Autodesk Inventor part; units mm, degrees
ref_plane "YZ Plane" through (0, 0, 0) normal (1, 0, 0) x (0, 1, 0)
ref_plane "XZ Plane" through (0, 0, 0) normal (0, 1, 0) x (-1, 0, 0)
ref_plane "XY Plane" through (0, 0, 0) normal (0, 0, 1) x (1, 0, 0)
sketch "Sketch1" plane through (0, 0, 0) normal (0, 0, 1) x (1, 0, 0)
  line L0 (0, 0) -> (5, 0)
  line L1 (5, 0) -> (5, 22)
  line L2 (5, 22) -> (0, 22)
  line L3 (0, 22) -> (0, 0)
  line L4 (2.5, 0) -> (2.5, 22) construction
  circle A0 centre (2.5, 13.75) radius 1.575
  line L5 (4, 2.25) -> (1, 2.25)
  line L6 (1, 2.25) -> (1, 9.25)
  line L7 (1, 9.25) -> (4, 9.25)
  line L8 (4, 9.25) -> (4, 2.25)
  dimension "d0" = 5
  dimension "d1" = 22
  dimension "d2" = 3.15
  dimension "d3" = 13.75
  dimension "d7" = 7
  dimension "d8" = 2.25
  dimension "d9" = 1
  dimension "d10" = 1
extrude "Extrusion1" add sketch "Sketch1" along normal blind 10
fillet "Fillet1" radius 1 8 edges at (2.5, 22, 10) (5, 11, 10) (2.5, 0, 10) (5, 22, 5) (0, 22, 5) (5, 0, 5) (0, 0, 5) (0, 11, 10)
sketch "Sketch2" plane through (0, 0, 0) normal (0, 0, -1) x (-1, 0, 0)
  line L0 (-1, 0) -> (-4, 0)
  line L1 (0, 21) -> (0, 1)
  line L2 (-4, 22) -> (-1, 22)
  line L3 (-5, 1) -> (-5, 21)
  line L4 (-1, 9.25) -> (-1, 2.25)
  line L5 (-1, 2.25) -> (-4, 2.25)
  line L6 (-4, 2.25) -> (-4, 9.25)
  line L7 (-4, 9.25) -> (-1, 9.25)
  circle A0 centre (-2.5, 13.75) radius 1.575
  arc A1 (-5, 1) -> (-4, 0) centre (-4, 1) ccw
  arc A2 (-1, 0) -> (0, 1) centre (-1, 1) ccw
  arc A3 (0, 21) -> (-1, 22) centre (-1, 21) ccw
  arc A4 (-4, 22) -> (-5, 21) centre (-4, 21) ccw
  point P0 (0, 0)
extrude "Extrusion2" add sketch "Sketch2" against normal blind 2.5 contours L4 L5 L6 L7
sketch "Sketch4" plane through (0, 0, 0) normal (0, -1, 0) x (1, 0, 0)
  line L0 (1, 0) -> (4, 0)
  line L1 (1, 10) -> (4, 10) construction
  line L2 (2.5, 10) -> (2.5, 0) construction
  line L3 (4.075, 0) -> (0.925, 0) construction
  circle A0 centre (2.5, 5) radius 1
  line L4 (4, 9) -> (4, 0)
  line L5 (1, 9) -> (4, 9)
  line L6 (1, 0) -> (1, 9)
  point P0 (0, 0)
  dimension "d13" = 2
  dimension "d14" = 5
extrude "Extrusion3" cut sketch "Sketch4" against normal blind 10.5 contours A0
chamfer "Chamfer1" distance 1 angle 45 1 edges at (1.5, 0, 5)
equation "\"d10\" = d9"
properties part number "hotend__belt_holder" material "ABS Plastic"
Build history of the part. All positions in model axes, mm. A direction names the side the tool comes from. Round coordinates to 2 decimals unless told otherwise and drop trailing zeros. Order: outer loops, then holes, each group sorted by start corner. A loop starts at its lowest first (then second) coordinate and runs counter-clockwise, first axis right, second up. Notation, with made-up numbers: (40, -17.5) -> (88, -17.5) arc R22 cw to (88, -0.5) -> close; hole circle Ø10 at (-34.5, 73.5). An arc over 180 degrees is marked (long way). Answer in a Markdown table with one row per item.
1) Mould opens along Y. For faces 4 (the cylindrical face through (0.285, 0.301, 4.563)), 5 (the flat face through (2.5, 2.25, 6.2)), 6 (the cylindrical face through (0.301, 17.568, 9.715)) say: released by +Y, released by -Y, zero draft, split by the parting line, or undercut.
Values:
| item | result |
|---|---|
| face 4 | released by -Y |
| face 5 | undercut |
| face 6 | zero draft |
2) Wall check: L1, parallel to X at y = 13.75, z = 7 (3 decimals); L2, parallel to Z at x = 2.5, y = 10.25; L3, parallel to X at y = 4.5, z = 2.75. Give the ranges that are in metal, low to high.
Values:
| item | result |
|---|---|
| L1 | 0 to 0.925, 4.075 to 5 |
| L2 | 0 to 4, 6 to 10 |
| L3 | 0 to 1, 4 to 5 |
3) Which spindle directions (+Z, -Z, +X, -X, +Y, -Y) get a long thin tool onto all of the face, cutting with end or side? Do faces 1 (the cylindrical face through (1.763, 9.866, 5.676)), 2 (the flat face through (2.5, 9.25, 6.2)), 3 (the cylindrical face through (4.715, 21.699, 4.563)). Say none if no direction does.
Values:
| item | result |
|---|---|
| face 1 | -Y |
| face 2 | +Z |
| face 3 | +Z, -Z, +X, +Y |
4) Band-saw the part on D-D on z = 5. Give the cut face in (x, y) (3 decimals).
Values:
| item | result |
|---|---|
| outline | (0, 1) arc R1 ccw to (0.589, 0.089) -> (1.5, 1) -> (1.5, 2.25) -> (1, 2.25) -> (1, 9.25) -> (1.5, 9.25) -> (1.5, 10.5) -> (3.5, 10.5) -> (3.5, 9.25) -> (4, 9.25) -> (4, 2.25) -> (3.5, 2.25) -> (3.5, 1) -> (4.411, 0.089) arc R1 ccw to (5, 1) -> (5, 21) arc R1 ccw to (4, 22) -> (1, 22) arc R1 ccw to (0, 21) -> close; hole circle Ø3.15 at (2.5, 13.75) |
5) Pin check, flat tips, straight feed: P1, Ø1.6, axis at x = 2.5, z = 5, coming from the -Y side; P2, Ø2, axis at x = 3, z = 5, coming from the -Y side; P3, Ø2, axis at x = 2.5, y = 6.5, coming from the +Z side. Stop position of each tip, or through.
Values:
| item | result |
|---|---|
| P1 | y = 10.5 |
| P2 | y = 0.5 |
| P3 | z = 2.5 |
6) Band-saw the part on B-B on z = 7.75. Give the cut face in (x, y) (3 decimals).
Values:
| item | result |
|---|---|
| outline | (0, 1) arc R1 ccw to (1, 0) -> (4, 0) arc R1 ccw to (5, 1) -> (5, 21) arc R1 ccw to (4, 22) -> (1, 22) arc R1 ccw to (0, 21) -> close; hole circle Ø3.15 at (2.5, 13.75); hole (1, 2.25) -> (4, 2.25) -> (4, 9.25) -> (1, 9.25) -> close |
7) Band-saw the part on A-A on x = 2.5. Give the cut face in (y, z) (3 decimals), and give its area (3 significant figures).
Values:
| item | result |
|---|---|
| outline | (0, 0) -> (12.175, 0) -> (12.175, 10) -> (9.25, 10) -> (9.25, 6) -> (10.5, 6) -> (10.5, 4) -> (9.25, 4) -> (9.25, 2.5) -> (2.25, 2.5) -> (2.25, 4) -> (1, 4) -> (0, 3) -> close; (0, 7) -> (1, 6) -> (2.25, 6) -> (2.25, 10) -> (1, 10) arc R1 ccw to (0, 9) -> close; (15.325, 0) -> (22, 0) -> (22, 9) arc R1 ccw to (21, 10) -> (15.325, 10) -> close |
| area | 128 mm2 |
